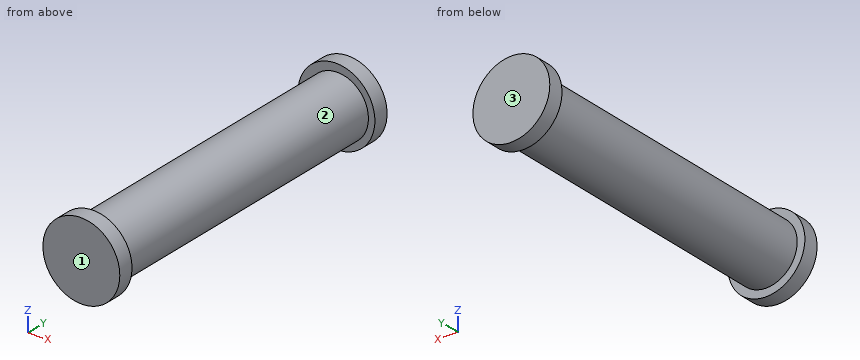
```python
from build123d import *

# Parameters (mm, degrees)
F0_R     = 4
F1_DEPTH = 40
F2_R     = 5
F2_R_2   = 4
F3_DEPTH = 2
F4_R     = 5
F4_R_2   = 4
F5_DEPTH = 2


with BuildPart() as f1:
    # F0 (on Front) → F1 (new body)
    with BuildSketch(Plane.XZ):
        Circle(F0_R)
    extrude(amount=F1_DEPTH)

    # F2 (on face) → F3 (join)
    with BuildSketch(Plane.XZ.offset(40)):
        Circle(F2_R)
        Circle(F2_R_2, mode=Mode.SUBTRACT)
        Circle(F2_R_2)
    extrude(amount=F3_DEPTH)

    # F4 (on face) → F5 (join)
    with BuildSketch(Plane(origin=(0, 0, 0), x_dir=(-1, 0, 0), z_dir=(0, 1, 0))):
        with Locations((0.1622709678, 0)):
            Circle(F4_R)
        Circle(F4_R_2, mode=Mode.SUBTRACT)
        Circle(F4_R_2)
    extrude(amount=F5_DEPTH)


solid = f1.part
```
For this review, take the finished solid that the model builds, in its own axes (mm). Face numbers are marked on the shaded views. Give positions to 0.01 mm unless a question says otherwise; leave off trailing zeros. Write each loop counter-clockwise with the first axis right and the second up, starting at its lowest first coordinate (ties: lowest second). Pieces come first, ordered by that corner, then holes.
Item 1: Take a section at A-A (z = 0). Give the boundary of the cut face in (x, y), and give its area (3 significant figures).
Item 2: Wall thickness on probe 1 along Y at (x, z) = (3.75, -2); probe 2 along Z at (x, y) = (2.75, -39); probe 3 along X at (y, z) = (-18.5, -0.5): over which ranges is each line inside the solid? List them lowest first.
Item 3: Take a section at B-B (x = 3.25). Give the boundary of the cut face in (y, z), and give its area (3 significant figures).
Item 4: The part is to be moulded in two halves that separate along Y. For the marked faces 1, 2 and 3, say which applies: +Y half, -Y half, draft (parallel to the pull), parting line (faces both ways), or undercut.
Item 5: Take a section at C-C (y = -33). Give the boundary of the cut face in (x, z).
Item 6: Insertion check: P1, Ø5, axis at x = 1.5, y = -30.5, coming from the -Z side; P2, Ø1, axis at y = -3.5, z = 1, coming from the +X side; P3, Ø3, axis at y = -29, z = 1.5, coming from the -X side. Each pin has a flat end and moves straight along its axis. Give the tip position at first contact, or say it passes through.
Established:
1. outline: (-5.16, 0) - (-4, 0) - (-4, -40) - (-5, -40) - (-5, -42) - (5, -42) - (5, -40) - (4, -40) - (4, 0) - (4.84, 0) - (4.84, 2) - (-5.16, 2) - close
1. area: 360 mm2
2. probe 1: y = -42 to -40, 0 to 2
2. probe 2: z = -2.9 to 2.9
2. probe 3: x = -3.97 to 3.97
3. outline: (-42, -3.8) - (-40, -3.8) - (-40, -2.33) - (0, -2.33) - (0, -3.65) - (2, -3.65) - (2, 3.65) - (0, 3.65) - (0, 2.33) - (-40, 2.33) - (-40, 3.8) - (-42, 3.8) - close
3. area: 216 mm2
4. face 1: -Y half
4. face 2: undercut
4. face 3: +Y half
5. outline: circle Ø8 at (0, 0)
6. P1: stops at z = -4
6. P2: stops at x = 3.97
6. P3: stops at x = -4
